Check sheet for the modelled part. Datum: model origin and axes. Units: mm. Face numbers are marked on the shaded views. A direction names the side the tool comes from. Round coordinates to 2 decimals unless told otherwise and drop trailing zeros. Loops run counter-clockwise (first coordinate to the right, second up) from the corner with the lowest first, then second, coordinate; pieces in that order, holes last. Notation, with made-up numbers: (54.25, -4.5) - (66.25, -4.5) arc R10 ccw to (66.25, 8.5) - close; hole circle Ø6 at (25.5, -12.75). An arc over 180 degrees is marked (long way). Return JSON: item names as keys, results as strings.
from build123d import *

# Parameters (mm, degrees)
AUFSATZ_LINEAR_AUSTRAGEN1_DEPTH      = 4
AUFSATZ_LINEAR_AUSTRAGEN1_2_DEPTH    = 4
AUFSATZ_LINEAR_AUSTRAGEN1_3_DEPTH    = 4
AUFSATZ_LINEAR_AUSTRAGEN1_4_DEPTH    = 4
SKIZZE2_R                            = 27.1
AUFSATZ_LINEAR_AUSTRAGEN2_DEPTH      = 2
AUFSATZ_LINEAR_AUSTRAGEN3_DEPTH      = 4
AUFSATZ_LINEAR_AUSTRAGEN4_DEPTH      = 10.258635
KREISMUSTER3_COUNT                   = 4
AUFSATZ_LINEAR_AUSTRAGEN5_DEPTH      = 2
SCHNITT_LINEAR_AUSTRAGEN1_DEPTH      = 1
SCHNITT_LINEAR_AUSTRAGEN1_DEPTH_BACK = 101
SKIZZE11_W                           = 40
SKIZZE11_H                           = 80
SKIZZE11_W_2                         = 36
SKIZZE11_H_2                         = 76
AUFSATZ_LINEAR_AUSTRAGEN6_DEPTH      = 10
AUFSATZ_LINEAR_AUSTRAGEN7_REACH      = 85.898
SKIZZE12_W                           = 7.5
SKIZZE12_H                           = 3
SCHNITT_LINEAR_AUSTRAGEN2_DEPTH      = 1.0000001
SCHNITT_LINEAR_AUSTRAGEN2_DEPTH_BACK = 101.0000001
SKIZZE14_R                           = 5
AUFSATZ_LINEAR_AUSTRAGEN8_DEPTH      = 20
KERNLOCH_F_R_M4_GEWINDE1_D           = 3.3
KERNLOCH_F_R_M4_GEWINDE1_DEPTH       = 20
KERNLOCH_F_R_M4_GEWINDE1_TIP         = 0.991420021


with BuildPart() as part:
    # Skizze1 → Aufsatz-Linear austragen1 (new body)
    with BuildSketch(Plane.XY):
        with BuildLine():
            Line((-6, -24.372320366), (-6, -26.427447853))
            ThreePointArc((-6, -26.427447853), (-19.16259377, -19.16259377), (-26.427447853, -6))
            Line((-26.427447853, -6), (-24.372320366, -6))
            ThreePointArc((-24.372320366, -6), (-17.748380208, -17.748380208), (-6, -24.372320366))
        make_face()
    extrude(amount=AUFSATZ_LINEAR_AUSTRAGEN1_DEPTH)



with BuildPart() as body_2:
    # Skizze1 → Aufsatz-Linear austragen1 2 (new body)
    with BuildSketch(Plane.XY):
        with BuildLine():
            Line((6, -24.372320366), (6, -26.427447853))
            ThreePointArc((6, -26.427447853), (19.16259377, -19.16259377), (26.427447853, -6))
            Line((26.427447853, -6), (24.372320366, -6))
            ThreePointArc((24.372320366, -6), (17.748380208, -17.748380208), (6, -24.372320366))
        make_face()
    extrude(amount=AUFSATZ_LINEAR_AUSTRAGEN1_2_DEPTH)


with BuildPart() as body_3:
    # Skizze1 → Aufsatz-Linear austragen1 3 (new body)
    with BuildSketch(Plane.XY):
        with BuildLine():
            Line((-24.372320366, 6), (-26.427447853, 6))
            ThreePointArc((-26.427447853, 6), (-19.16259377, 19.16259377), (-6, 26.427447853))
            Line((-6, 26.427447853), (-6, 24.372320366))
            ThreePointArc((-6, 24.372320366), (-17.748380208, 17.748380208), (-24.372320366, 6))
        make_face()
    extrude(amount=AUFSATZ_LINEAR_AUSTRAGEN1_3_DEPTH)


with BuildPart() as body_4:
    # Skizze1 → Aufsatz-Linear austragen1 4 (new body)
    with BuildSketch(Plane.XY):
        with BuildLine():
            Line((6, 24.372320366), (6, 26.427447853))
            ThreePointArc((6, 26.427447853), (19.16259377, 19.16259377), (26.427447853, 6))
            Line((26.427447853, 6), (24.372320366, 6))
            ThreePointArc((24.372320366, 6), (17.748380208, 17.748380208), (6, 24.372320366))
        make_face()
    extrude(amount=AUFSATZ_LINEAR_AUSTRAGEN1_4_DEPTH)


with BuildPart() as part_1:
    add(part.part)

    add(body_2.part)  # Aufsatz-Linear austragen2 merges body 2

    add(body_3.part)  # Aufsatz-Linear austragen2 merges body 3

    add(body_4.part)  # Aufsatz-Linear austragen2 merges body 4
    # Skizze2 → Aufsatz-Linear austragen2 (add)
    with BuildSketch(Plane(origin=(0, 0, 0), x_dir=(-1, 0, 0), z_dir=(0, 0, -1))):
        Circle(SKIZZE2_R)
    extrude(amount=AUFSATZ_LINEAR_AUSTRAGEN2_DEPTH)


with BuildPart() as body_2_2:
    # Skizze3 → Aufsatz-Linear austragen3 (new body)
    with BuildSketch(Plane.XY):
        with BuildLine():
            Line((5.129317712, -26.610150315), (5.129317712, -25.1))
            Line((5.129317712, -25.1), (0, -25.1))
            Line((0, -25.1), (-5.129317712, -25.1))
            Line((-5.129317712, -25.1), (-5.129317712, -26.610150315))
            ThreePointArc((-5.129317712, -26.610150315), (0, -27.1), (5.129317712, -26.610150315))
        make_face()
    extrude(amount=AUFSATZ_LINEAR_AUSTRAGEN3_DEPTH)


with BuildPart() as body_3_2:
    # Skizze4 → Aufsatz-Linear austragen4 (new body)
    with BuildSketch(Plane.ZY.offset(5.129317712)):
        Polygon((4, -25.1), (3, -24.1), (2.8, -24.1), (2.8, -25.1), align=None)
    extrude(amount=-AUFSATZ_LINEAR_AUSTRAGEN4_DEPTH)


with BuildPart() as kreismuster3_1:
    # Kreismuster3: pattern copy
    add(body_3_2.part.rotate(Axis((0, 0, 0), (0, 0, 1)), 1 * 360 / KREISMUSTER3_COUNT))


with BuildPart() as kreismuster3_2:
    # Kreismuster3: pattern copy
    add(body_3_2.part.rotate(Axis((0, 0, 0), (0, 0, 1)), 2 * 360 / KREISMUSTER3_COUNT))


with BuildPart() as kreismuster3_3:
    # Kreismuster3: pattern copy
    add(body_3_2.part.rotate(Axis((0, 0, 0), (0, 0, 1)), 3 * 360 / KREISMUSTER3_COUNT))


with BuildPart() as kreismuster3_4:
    # Kreismuster3: pattern copy
    add(body_2_2.part.rotate(Axis((0, 0, 0), (0, 0, 1)), 1 * 360 / KREISMUSTER3_COUNT))


with BuildPart() as kreismuster3_5:
    # Kreismuster3: pattern copy
    add(body_2_2.part.rotate(Axis((0, 0, 0), (0, 0, 1)), 2 * 360 / KREISMUSTER3_COUNT))


with BuildPart() as kreismuster3_6:
    # Kreismuster3: pattern copy
    add(body_2_2.part.rotate(Axis((0, 0, 0), (0, 0, 1)), 3 * 360 / KREISMUSTER3_COUNT))


with BuildPart() as part_2:
    add(part_1.part)

    # Kombinieren1: union Kreismuster3_6, Kreismuster3_5, Kreismuster3_4, body 2 2, Kreismuster3_3, Kreismuster3_2, Kreismuster3_1, body 3 2
    add(kreismuster3_6.part)
    add(kreismuster3_5.part)
    add(kreismuster3_4.part)
    add(body_2_2.part)
    add(kreismuster3_3.part)
    add(kreismuster3_2.part)
    add(kreismuster3_1.part)
    add(body_3_2.part)

    # Skizze5 → Aufsatz-Linear austragen5 (add)
    with BuildSketch(Plane(origin=(0, 0, -2), x_dir=(-1, 0, 0), z_dir=(0, 0, -1))):
        with BuildLine():
            Line((30, 75), (-30, 75))
            ThreePointArc((-30, 75), (-44.142135624, 69.142135624), (-50, 55))
            Line((-50, 55), (-50, -55))
            ThreePointArc((-50, -55), (-44.142135624, -69.142135624), (-30, -75))
            Line((-30, -75), (30, -75))
            ThreePointArc((30, -75), (44.142135624, -69.142135624), (50, -55))
            Line((50, -55), (50, 55))
            ThreePointArc((50, 55), (44.142135624, 69.142135624), (30, 75))
        make_face()
    extrude(amount=AUFSATZ_LINEAR_AUSTRAGEN5_DEPTH)

    # Austragung2: sweep along a path in Skizze7
    with BuildLine(Plane(origin=(0, 0, 0), x_dir=(0, 0, -1), z_dir=(1, 0, 0))) as austragung2_path:
        Line((2, 75), (-91.969262079, 109.202014333))
    # Skizze6 → Austragung2 (sweep)
    with BuildSketch(Plane.XY.offset(-2)):
        with BuildLine():
            Line((50, -55), (50, 55))
            ThreePointArc((50, 55), (44.142135624, 69.142135624), (30, 75))
            Line((30, 75), (-30, 75))
            ThreePointArc((-30, 75), (-44.142135624, 69.142135624), (-50, 55))
            Line((-50, 55), (-50, -55))
            ThreePointArc((-50, -55), (-44.142135624, -69.142135624), (-30, -75))
            Line((-30, -75), (30, -75))
            ThreePointArc((30, -75), (44.142135624, -69.142135624), (50, -55))
        make_face()
        with BuildLine():
            Line((48, -55), (48, 55))
            ThreePointArc((48, 55), (42.727922061, 67.727922061), (30, 73))
            Line((30, 73), (-30, 73))
            ThreePointArc((-30, 73), (-42.727922061, 67.727922061), (-48, 55))
            Line((-48, 55), (-48, -55))
            ThreePointArc((-48, -55), (-42.727922061, -67.727922061), (-30, -73))
            Line((-30, -73), (30, -73))
            ThreePointArc((30, -73), (42.727922061, -67.727922061), (48, -55))
        make_face(mode=Mode.SUBTRACT)
    sweep(path=austragung2_path.line)

    # Skizze8 → Schnitt-Linear austragen1 (cut, two sides)
    with BuildSketch(Plane(origin=(50, 0, 0), x_dir=(0, 0, -1), z_dir=(1, 0, 0))) as schnitt_linear_austragen1_sk:
        Polygon((-91.969262079, -20.797985667), (-82.427373137, -24.270949221), (-29.94698396, 66.627751236), (-91.969262079, 89.202014333), align=None)
        Polygon((-91.969262079, 89.202014333), (-29.94698396, 66.627751236), (-20.405095018, 83.154787683), (-91.969262079, 109.202014333), align=None)
        Polygon((-91.969262079, -20.797985667), (-91.969262079, -40.797985667), (-82.427373137, -24.270949221), align=None)
    extrude(amount=SCHNITT_LINEAR_AUSTRAGEN1_DEPTH, mode=Mode.SUBTRACT)
    extrude(schnitt_linear_austragen1_sk.sketch, amount=-SCHNITT_LINEAR_AUSTRAGEN1_DEPTH_BACK, mode=Mode.SUBTRACT)

    # Skizze11 → Aufsatz-Linear austragen6 (add)
    with BuildSketch(Plane(origin=(0, -63.817834564, 23.227792197), x_dir=(1, 0, 0), z_dir=(0, 0.939692621, -0.342020143))):
        with Locations((0, -13.153144296)):
            Rectangle(SKIZZE11_W, SKIZZE11_H)
        with Locations((0, -13.153144296)):
            Rectangle(SKIZZE11_W_2, SKIZZE11_H_2, mode=Mode.SUBTRACT)
    extrude(amount=AUFSATZ_LINEAR_AUSTRAGEN6_DEPTH)

    # Aufsatz-Linear austragen7: up to this face of the body (flat: up to its plane)
    aufsatz_linear_austragen7_end = Plane(part_2.part.faces().sort_by_distance((0, 0.797060642, -4))[0])
    # Skizze12 → Aufsatz-Linear austragen7 (add, up to the picked face)
    with BuildSketch(Plane(origin=(0, 18.17944603, 49.947617466), x_dir=(1, 0, 0), z_dir=(0, 0.342020143, 0.939692621)), mode=Mode.PRIVATE) as aufsatz_linear_austragen7_sk1:
        with Locations((-3.75, -59.413521031)):
            Rectangle(SKIZZE12_W, SKIZZE12_H)
    aufsatz_linear_austragen7_tool1 = split(extrude(aufsatz_linear_austragen7_sk1.sketch, amount=-AUFSATZ_LINEAR_AUSTRAGEN7_REACH, mode=Mode.PRIVATE), bisect_by=aufsatz_linear_austragen7_end, keep=Keep.BOTH, mode=Mode.PRIVATE)
    add(aufsatz_linear_austragen7_tool1.solids().sort_by_distance((-3.75, -37.651001, 70.268238))[0])
    # Skizze12 → Aufsatz-Linear austragen7 (add, up to the picked face)
    with BuildSketch(Plane(origin=(0, 18.17944603, 49.947617466), x_dir=(1, 0, 0), z_dir=(0, 0.342020143, 0.939692621)), mode=Mode.PRIVATE) as aufsatz_linear_austragen7_sk2:
        with Locations((3.75, -59.413521031)):
            Rectangle(SKIZZE12_W, SKIZZE12_H)
    aufsatz_linear_austragen7_tool2 = split(extrude(aufsatz_linear_austragen7_sk2.sketch, amount=-AUFSATZ_LINEAR_AUSTRAGEN7_REACH, mode=Mode.PRIVATE), bisect_by=aufsatz_linear_austragen7_end, keep=Keep.BOTH, mode=Mode.PRIVATE)
    add(aufsatz_linear_austragen7_tool2.solids().sort_by_distance((3.75, -37.651001, 70.268238))[0])

    # Skizze13 → Schnitt-Linear austragen2 (cut, two sides)
    with BuildSketch(Plane(origin=(50, 0, 0), x_dir=(0, 0, -1), z_dir=(1, 0, 0))) as schnitt_linear_austragen2_sk:
        Polygon((4, -47.000472849), (4, -75), (25.669622084, -47.000472849), align=None)
    extrude(amount=SCHNITT_LINEAR_AUSTRAGEN2_DEPTH, mode=Mode.SUBTRACT)
    extrude(schnitt_linear_austragen2_sk.sketch, amount=-SCHNITT_LINEAR_AUSTRAGEN2_DEPTH_BACK, mode=Mode.SUBTRACT)

    # Skizze14 → Aufsatz-Linear austragen8 (add)
    with BuildSketch(Plane(origin=(0, -99.846855704, -2), x_dir=(1, 0, 0), z_dir=(0, 0, 1))):
        with Locations((-20, 69.846855704)):
            Circle(SKIZZE14_R)
        with Locations((20, 69.846855704)):
            Circle(SKIZZE14_R)
        with Locations((-20, 129.846855704)):
            Circle(SKIZZE14_R)
        with Locations((20, 129.846855704)):
            Circle(SKIZZE14_R)
    extrude(amount=AUFSATZ_LINEAR_AUSTRAGEN8_DEPTH)

    # Kernloch für M4 Gewinde1
    with Locations(Plane.XY.offset(18)):
        with Locations((-20, 30), (20, 30), (20, -30), (-20, -30)):
            Hole(KERNLOCH_F_R_M4_GEWINDE1_D / 2, depth=KERNLOCH_F_R_M4_GEWINDE1_DEPTH)
            with Locations((0, 0, -(KERNLOCH_F_R_M4_GEWINDE1_DEPTH + KERNLOCH_F_R_M4_GEWINDE1_TIP / 2))):  # 118° drill point
                Cone(0, KERNLOCH_F_R_M4_GEWINDE1_D / 2, KERNLOCH_F_R_M4_GEWINDE1_TIP, mode=Mode.SUBTRACT)


solid = part_2.part
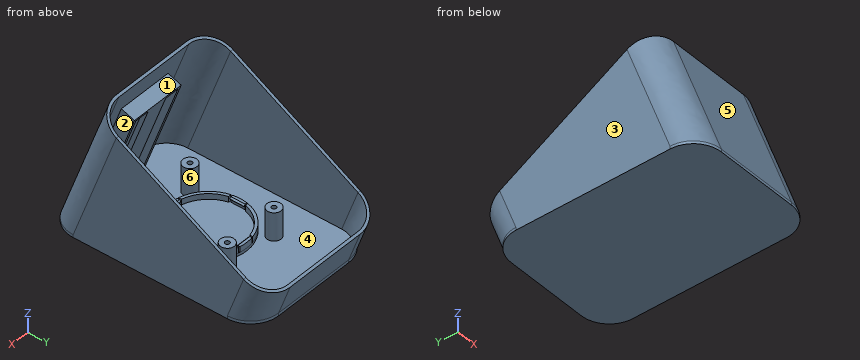
Q1. Scan lines: probe 1 along X at (y, z) = (-17.5, 43); probe 2 along X at (y, z) = (26.5, 7.5); probe 3 along Z at (x, y) = (-0.5, 29.5). Record each from-to range of solid material in increasing order. Write a range as [from, to].
Answer key:
{"probe 1": "x = [-50, -48], [48, 50]", "probe 2": "x = [-50, -48], [-23.57, -16.43], [16.43, 23.57], [48, 50]", "probe 3": "z = [-4, -2]"}
Q2. Draft check along Y on the marked faces 1, 2 and 3. Enter one of: released by +Y, released by -Y, zero draft, split by the parting line, or undercut.
Answer key:
{"face 1": "released by +Y", "face 2": "undercut", "face 3": "zero draft"}
Q3. Tool access check on the marked faces 4, 5 and 6. Record the directions out of +Z, -Z, +X, -X, +Y, -Y that give a thin tool (end or side, any length) a straight path to the whole face; none if there is none.
Answer key:
{"face 4": "none", "face 5": "+Z, +X, -X, -Y", "face 6": "+Z"}
Q4. Depth check by flat-ended pin: P1, Ø1.2, axis at x = -26, z = 2, coming from the -Y side; P2, Ø8, axis at x = -22, y = 29.5, coming from the +Z side; P3, Ø2, axis at x = 26.5, y = -2.5, coming from the +Z side. Enter the tip coordinate at first touch or a pass-through.
Answer key:
{"P1": "stops at y = -73.76", "P2": "stops at z = 18", "P3": "stops at z = 4"}
Q5. Sectioned sample at A-A (y = 0). Enter the section's corners in (x, z), plus the area to 3 significant figures.
Answer key:
{"outline": "(-50, -4) - (50, -4) - (50, 68.41) - (48, 68.41) - (48, -2) - (27.1, -2) - (27.1, 4) - (25.1, 4) - (24.1, 3) - (24.1, 2.8) - (25.1, 2.8) - (25.1, 0) - (-25.1, 0) - (-25.1, 2.8) - (-24.1, 2.8) - (-24.1, 3) - (-25.1, 4) - (-27.1, 4) - (-27.1, -2) - (-48, -2) - (-48, 68.41) - (-50, 68.41) - close", "area": "607 mm²"}
